from build123d import *

# Parameters (mm, degrees)
F1_DEPTH        = 101.6
F2_T            = -1.5748
F4_DEPTH        = 101.6
F4_COPIES_COUNT = 4
F6_W            = 50.8
F6_H            = 25.4
F7_DEPTH        = 1.5748
F7_COPIES_COUNT = 4


# Not quite as in the source:
# - a pattern or mirror of a feature is missing from the dataset's text; its kind, count and spacing are read off the source's solid


with BuildPart() as f1:
    # F0 (on Top) → F1 (new body)
    with BuildSketch(Plane.XY):
        Polygon((76.3321770291, 0), (0, 76.3321770291), (-76.3321770291, 0), (0, -76.3321770291), align=None)
    extrude(amount=F1_DEPTH)

    # F2
    f2_openings = [f1.faces().sort_by_distance(p)[0] for p in [
        (0, 0, 101.6),
        (0, 0, 0),
    ]]
    offset(amount=F2_T, openings=f2_openings)

    # F3 (on face) → F4 (join, through all)
    with BuildSketch(Plane.XY.offset(101.6)):
        Polygon((-101.6, -0.7874), (-75.5447770291, -0.7874), (-76.3321770291, 0), (-75.5447770291, 0.7874), (-101.6, 0.7874), align=None)
        Polygon((-75.5447770291, -0.7874), (-73.3176735111, -0.7874), (-74.1050735111, 0), (-73.3176735111, 0.7874), (-75.5447770291, 0.7874), (-76.3321770291, 0), align=None)
    f4 = extrude(amount=-F4_DEPTH)

    # F4_copies: F4 ×4 about axis
    f4_copies_axis = Axis((0, 0, 0), (0, 0, 1))
    for i in range(1, F4_COPIES_COUNT):
        add(f4.rotate(f4_copies_axis, i * 360 / F4_COPIES_COUNT))

    # F6 (on face) → F7 (cut, through all)
    with BuildSketch(Plane(origin=(38.1660885145, -38.1660885145, 0), x_dir=(0.7071067812, 0.7071067812, 0), z_dir=(0.7071067812, -0.7071067812, 0))):
        with Locations((0, 12.7)):
            Rectangle(F6_W, F6_H)
    f7 = extrude(amount=-F7_DEPTH, mode=Mode.SUBTRACT)

    # F7_copies: F7 ×4 about axis
    f7_copies_axis = Axis((0, 0, 0), (0, 0, 1))
    for i in range(1, F7_COPIES_COUNT):
        add(f7.rotate(f7_copies_axis, i * 360 / F7_COPIES_COUNT), mode=Mode.SUBTRACT)


solid = f1.part
Verification items for the finished model (mm, model axes). A direction names the side the tool comes from. Coordinates: 2 decimals unless noted, no trailing zeros. Loops run counter-clockwise (first coordinate to the right, second up) from the corner with the lowest first, then second, coordinate; pieces in that order, holes last. Notation, with made-up numbers: M -4,70 L 10,70 A28 cw 10,108 Z; hole C -32.5,-34 d8. An arc over 180 degrees is marked long. One line per item, written item: value.
1. Section check B-B on y = 68.5. Record the cut outline in (x, z), plus the area to 3 significant figures.
Answers follow:
outline: M -7.83,0 L -5.61,0 L -5.61,101.6 L -7.83,101.6 Z; M 5.61,0 L 7.83,0 L 7.83,101.6 L 5.61,101.6 Z
area: 453 mm^2
2. Material ranges on line 1 along X through (y, z) = (80.5, 14); line 2 along Y through (x, z) = (-50, 94.5), recorded low to high. Write a range as from..to.
Answers follow:
line 1: -0.79..0.79
line 2: -26.33..-24.11, 24.11..26.33
3. Set-up check for faces 1 (the flat face through (89, 0.787, 52)), 2 (the flat face through (88, -0.787, 52)), 3 (the flat face through (-0.787, -88, 52)): record each of +Z, -Z, +X, -X, +Y, -Y from which the full face is reachable in a straight line by a thin tool's end or side.
Answers follow:
face 1: +Z, -Z, +X, +Y
face 2: +Z, -Z, +X, -Y
face 3: +Z, -Z, -X, -Y
4. Section check A-A on x = 11.5. Record the cut outline in (y, z).
Answers follow:
outline: M -64.83,0 L -62.61,0 L -62.61,101.6 L -64.83,101.6 Z; M 62.61,0 L 64.83,0 L 64.83,101.6 L 62.61,101.6 Z
5. Gauge pin test, flat ends, axial feed: P1, Ø12, axis at x = 47.5, y = 29, coming from the -Z side; P2, Ø21, axis at x = 93, z = 73.5, coming from the -Y side; P3, Ø18.5, axis at x = -29, y = 29.5, coming from the -Z side; P4, Ø6, axis at x = 66.5, z = 55, coming from the +Y side. Record the tip position at first contact, or that the pin passes through.
Answers follow:
P1: z = 25.4
P2: y = -0.79
P3: through
P4: y = 12.83
6. Section check D-D on z = 16. Give the number of separate pieces and of enclosed holes in the cut face, plus the area to 3 significant figures.
Answers follow:
separate pieces: 4
enclosed holes: 0
area: 512 mm^2
7. Section check C-C on z = 77. Record the cut outline in (x, y), plus the area to 3 significant figures.
Answers follow:
outline: M -101.6,-0.79 L -75.54,-0.79 L -0.79,-75.54 L -0.79,-101.6 L 0.79,-101.6 L 0.79,-75.54 L 75.54,-0.79 L 101.6,-0.79 L 101.6,0.79 L 75.54,0.79 L 0.79,75.54 L 0.79,101.6 L -0.79,101.6 L -0.79,75.54 L -75.54,0.79 L -101.6,0.79 Z; hole M -74.11,0 L 0,-74.11 L 74.11,0 L 0,74.11 Z
area: 832 mm^2
